Check sheet for the modelled part. Datum: model origin and axes. Units: mm. Face numbers are marked on the shaded views. A direction names the side the tool comes from. Coordinates: 2 decimals unless noted, no trailing zeros. One line per item, written item: value. Start each with the question number.
1) Scan lines: line 1 along Y through (x, z) = (17.5, 16); line 2 along Z through (x, y) = (0.5, 63.5); line 3 along Z through (x, y) = (4.5, 7.5). Record each from-to range of solid material in increasing order. Write a range as [from, to].
2) Set-up check for the marked faces 3 and 4: record each of +Z, -Z, +X, -X, +Y, -Y from which the full face is reachable in a straight line by a thin tool's end or side.
3) Draft check along X on the marked faces 1 and 2. Enter one of: +X half, -X half, draft (parallel to the pull), parting line (faces both ways), or undercut.
4) Gauge pin test, flat ends, axial feed: P1, Ø1, axis at x = -1, z = -20.5, coming from the +Y side; P2, Ø10, axis at x = 11.5, y = 35, coming from the -Z side; P3, Ø2, axis at x = -23, y = 7.5, coming from the +Z side. Record the tip position at first contact, or that the pin passes through.
```python
from build123d import *

# Parameters (mm, degrees)
ESBO_O1_W                 = 50
ESBO_O1_H                 = 50
RESSALTO_EXTRUS_O1_DEPTH  = 41
RESSALTO_EXTRUS_O1_TAPER  = 2
FILETE1_R                 = 5
ESBO_O3_R                 = 1.25
CORTE_EXTRUS_O1_DEPTH     = 6
REVOLU_O2_ANGLE           = 10
REVOLU_O2_OTHER_WAY_ANGLE = 10
CORTE_EXTRUS_O2_DEPTH     = 5


with BuildPart() as part:
    # Esboço1 → Ressalto-extrusão1 (new body)
    with BuildSketch(Plane(origin=(0, 0, 0), x_dir=(1, 0, 0), z_dir=(0, 1, 0))):
        Rectangle(ESBO_O1_W, ESBO_O1_H)
    extrude(amount=RESSALTO_EXTRUS_O1_DEPTH, taper=RESSALTO_EXTRUS_O1_TAPER)

    # Esboço2 → Revolução1 (revolve)
    with BuildSketch(Plane(origin=(0, 0, 0), x_dir=(0, 0, -1), z_dir=(1, 0, 0))):
        Polygon((0, 41), (0, 70), (18.75, 70), (18.75, 61.5), (20, 54.5), (21, 54.5), (21, 41), align=None)
    revolve(axis=Axis((0, 41, 0), (0, 1, 0)))

    # Filete1
    filete1_edges = [part.edges().sort_by_distance(p)[0] for p in [
        (24.284124225, 20.5, 24.284124225),
        (-24.284124225, 20.5, 24.284124225),
        (-24.284124225, 20.5, -24.284124225),
        (24.284124225, 20.5, -24.284124225),
    ]]
    fillet(filete1_edges, radius=FILETE1_R)

    # Esboço3 → Corte-extrusão1 (cut)
    with BuildSketch(Plane(origin=(0, 0, 0), x_dir=(-1, 0, 0), z_dir=(0, -1, 0))):
        with Locations(Location((20, 20.625, 0), (0, 0, 90))):
            Circle(ESBO_O3_R)
        with Locations(Location((-20, -19.375, 0), (0, 0, 90))):
            Circle(ESBO_O3_R)
    extrude(amount=-CORTE_EXTRUS_O1_DEPTH, mode=Mode.SUBTRACT)

    # Esboço5 → Revolução2 (revolve)
    with BuildSketch(Plane(origin=(0, 0, 0), x_dir=(0, 0, -1), z_dir=(1, 0, 0))):
        Polygon((19.017857143, 60), (22, 60), (22, 41), (21, 41), (21, 54.5), (20, 54.5), align=None)
    revolve(axis=Axis((0, 41, 0), (0, -1, 0)), revolution_arc=REVOLU_O2_ANGLE)

    # Esboço5 → Revolução2 other way (revolve)
    with BuildSketch(Plane(origin=(0, 0, 0), x_dir=(0, 0, -1), z_dir=(1, 0, 0))):
        Polygon((19.017857143, 60), (22, 60), (22, 41), (21, 41), (21, 54.5), (20, 54.5), align=None)
    revolve(axis=Axis((0, 41, 0), (0, 1, 0)), revolution_arc=REVOLU_O2_OTHER_WAY_ANGLE)

    # Esboço7 → Corte-extrusão2 (cut)
    with BuildSketch(Plane(origin=(-25, 0, 0), x_dir=(0, 0, -1), z_dir=(1, 0, 0))):
        with BuildLine():
            Line((-16.1, 8.9), (-11.1, 8.9))
            ThreePointArc((-11.1, 8.9), (-10.392893219, 8.607106781), (-10.1, 7.9))
            Line((-10.1, 7.9), (-10.1, 5.9))
            ThreePointArc((-10.1, 5.9), (-10.392893219, 5.192893219), (-11.1, 4.9))
            Line((-11.1, 4.9), (-16.1, 4.9))
            ThreePointArc((-16.1, 4.9), (-16.807106781, 5.192893219), (-17.1, 5.9))
            Line((-17.1, 5.9), (-17.1, 7.9))
            ThreePointArc((-17.1, 7.9), (-16.807106781, 8.607106781), (-16.1, 8.9))
        make_face()
    extrude(amount=CORTE_EXTRUS_O2_DEPTH, mode=Mode.SUBTRACT)


solid = part.part
```
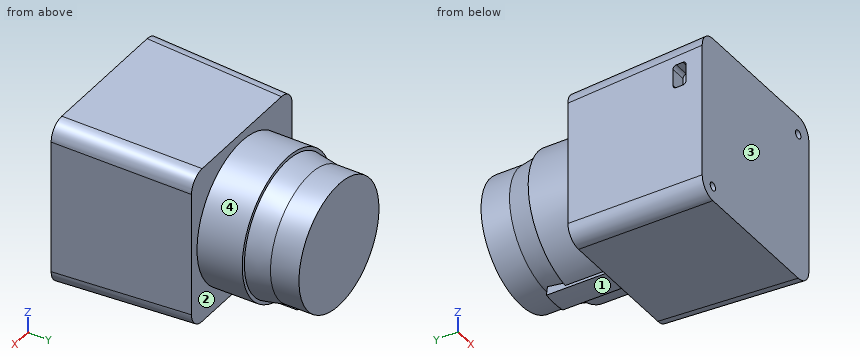
Answers:
1. line 1: y = [0, 41]
1. line 2: z = [-18.74, 18.74]
1. line 3: z = [-24.74, 24.74]
2. face 3: +Z, -Z, +X, -X, -Y
2. face 4: +Y
3. face 1: parting line
3. face 2: draft
4. P1: stops at y = 60
4. P2: stops at z = -23.95
4. P3: stops at z = 24.2
